Geometry: see drawing. Coordinates: mm, zero at the bounding-box minimum. Coordinates: 2 decimals unless noted, no trailing zeros. Order: outer loops, then holes, each group sorted by start corner. A loop starts at its lowest first (then second) coordinate and runs counter-clockwise, first axis right, second up. Notation, with made-up numbers: M -2.75,32.25 L 10.25,32.25 A8 ccw 10.25,37.25 Z; hole C 19,-38.5 d10. An arc over 180 degrees is marked long. Answer in a Markdown table with one row per item.
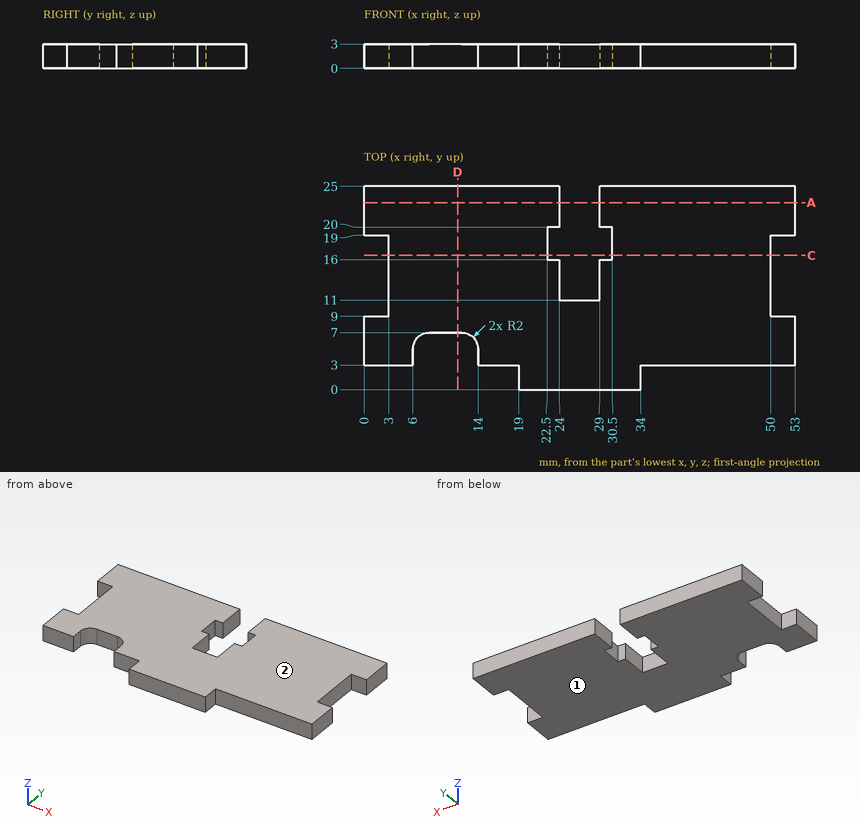
1) Mould query, pull axis Z, two halves, no side actions, for the marked faces 1 and 2. Classes: +Z half, -Z half, draft (parallel to the pull), parting line (faces both ways), or undercut.
Resolved:
| item | result |
|---|---|
| face 1 | -Z half |
| face 2 | +Z half |
2) Cut plane D-D, the plane x = 11.5. Output: boundary loops of the cut face in (y, z), and give its area (3 significant figures).
Resolved:
| item | result |
|---|---|
| outline | M 7,0 L 25,0 L 25,3 L 7,3 Z |
| area | 54.0 mm2 |
3) Material intervals for probe 1 along Y at (x, z) = (51, 0.2); probe 2 along X at (y, z) = (12.5, 0.6); probe 3 along X at (y, z) = (17.25, 0.6), sorted ascending.
Resolved:
| item | result |
|---|---|
| probe 1 | y = 3 to 9, 19 to 25 |
| probe 2 | x = 3 to 24, 29 to 50 |
| probe 3 | x = 3 to 22.5, 30.5 to 50 |
4) Cut plane A-A, the plane y = 23. Output: boundary loops of the cut face in (x, z), and give its area (3 significant figures).
Resolved:
| item | result |
|---|---|
| outline | M 0,0 L 24,0 L 24,3 L 0,3 Z; M 29,0 L 53,0 L 53,3 L 29,3 Z |
| area | 144 mm2 |
5) Contact query for flat-ended pins moving along their axis: pin 1 (1.5 mm diameter, centred on y = 1, z = 1.5, fed in from +X); pin 2 (0.9 mm diameter, centred on x = 47.5, z = 1.5, fed in from -Y). Output: stop coordinate, or through.
Resolved:
| item | result |
|---|---|
| pin 1 | stops at x = 34 |
| pin 2 | stops at y = 3 |
6) Cut plane C-C, the plane y = 16.5. Output: boundary loops of the cut face in (x, z).
Resolved:
| item | result |
|---|---|
| outline | M 3,0 L 22.5,0 L 22.5,3 L 3,3 Z; M 30.5,0 L 50,0 L 50,3 L 30.5,3 Z |
